```python
from build123d import *

# Parameters (mm, degrees)
BOSS_EXTRUDE1_DEPTH     = 3.175
CUT_EXTRUDE2_DEPTH      = 157.840117636
CUT_EXTRUDE2_DEPTH_BACK = 157.840117636
SKETCH3_R               = 1.25
CUT_EXTRUDE3_DEPTH      = 157.840117636
CUT_EXTRUDE3_DEPTH_BACK = 157.840117636
BOSS_EXTRUDE2_DEPTH     = 6.35
FILLET1_R               = 5
M6_CLEARANCE_HOLE1_D    = 6.6


with BuildPart() as part:
    # Sketch1 → Boss-Extrude1 (new, symmetric)
    with BuildSketch(Plane.XY):
        with BuildLine():
            Line((92.5, 126.5), (-92.5, 126.5))
            Line((-92.5, 126.5), (-92.5, 86.5))
            Line((-92.5, 86.5), (-42.012601066, -19.929660099))
            ThreePointArc((-42.012601066, -19.929660099), (0, -46.5), (42.012601066, -19.929660099))
            Line((42.012601066, -19.929660099), (92.5, 86.5))
            Line((92.5, 86.5), (92.5, 126.5))
        make_face()
    extrude(amount=BOSS_EXTRUDE1_DEPTH, both=True)

    # Sketch3 → Cut-Extrude2 (cut, two sides: drawn at the far end of the back side and taken through both)
    with BuildSketch(Plane(origin=(0, 0, -3.175), x_dir=(-1, 0, 0), z_dir=(0, 0, -1)).offset(-CUT_EXTRUDE2_DEPTH_BACK)):
        with Locations((17.440159599, -16.121517706)):
            Circle(SKETCH3_R)
        with Locations((22.282044228, -8.220280106)):
            Circle(SKETCH3_R)
        with Locations((9.943168767, -21.568400378)):
            Circle(SKETCH3_R)
        with Locations((0.932420624, -23.731689611)):
            Circle(SKETCH3_R)
        with Locations((-8.220280106, -22.282044228)):
            Circle(SKETCH3_R)
        with Locations((-16.121517706, -17.440159599)):
            Circle(SKETCH3_R)
        with Locations((-21.568400378, -9.943168767)):
            Circle(SKETCH3_R)
        with Locations((-23.731689611, -0.932420624)):
            Circle(SKETCH3_R)
        with Locations((-22.282044228, 8.220280106)):
            Circle(SKETCH3_R)
        with Locations((-17.440159599, 16.121517706)):
            Circle(SKETCH3_R)
        with Locations((-9.943168767, 21.568400378)):
            Circle(SKETCH3_R)
        with Locations((-0.932420624, 23.731689611)):
            Circle(SKETCH3_R)
        with Locations((8.220280106, 22.282044228)):
            Circle(SKETCH3_R)
        with Locations((16.121517706, 17.440159599)):
            Circle(SKETCH3_R)
        with Locations((21.568400378, 9.943168767)):
            Circle(SKETCH3_R)
        with Locations((23.731689611, 0.932420624)):
            Circle(SKETCH3_R)
    extrude(amount=CUT_EXTRUDE2_DEPTH + CUT_EXTRUDE2_DEPTH_BACK, mode=Mode.SUBTRACT)

    # Sketch4 → Cut-Extrude3 (cut, two sides: drawn at the far end of the back side and taken through both)
    with BuildSketch(Plane(origin=(0, 0, -3.175), x_dir=(-1, 0, 0), z_dir=(0, 0, -1)).offset(-CUT_EXTRUDE3_DEPTH_BACK)):
        with BuildLine():
            Line((-41.126950817, 21.698477285), (-73.85821292, 90.697419076))
            Line((-73.85821292, 90.697419076), (-73.85821292, 107.85821292))
            Line((-73.85821292, 107.85821292), (73.85821292, 107.85821292))
            Line((73.85821292, 107.85821292), (73.85821292, 90.697419076))
            Line((73.85821292, 90.697419076), (41.126950817, 21.698477285))
            ThreePointArc((41.126950817, 21.698477285), (0, 46.5), (-41.126950817, 21.698477285))
        make_face()
    extrude(amount=CUT_EXTRUDE3_DEPTH + CUT_EXTRUDE3_DEPTH_BACK, mode=Mode.SUBTRACT)

    # Sketch6 → Boss-Extrude2 (add)
    with BuildSketch(Plane.XY.offset(3.175)):
        Polygon((-32.71522073, 17.68327451), (0, 86.220686434), (32.71522073, 17.68327451), (49.538680905, 25.71368006), (10.328321936, 107.85821292), (-10.328321936, 107.85821292), (-49.538680905, 25.71368006), align=None)
    extrude(amount=-BOSS_EXTRUDE2_DEPTH)

    # Fillet1
    fillet1_edges = [part.edges().sort_by_distance(p)[0] for p in [
        (73.85821292, 90.697419076, 0),
        (73.85821292, 107.85821292, 0),
        (-73.85821292, 107.85821292, 0),
        (-73.85821292, 90.697419076, 0),
        (-46.275048201, 32.550893259, 0),
        (-21.466818467, 41.248341844, 0),
        (21.466818467, 41.248341844, 0),
        (0, 86.220686434, 0),
        (10.328321936, 107.85821292, 0),
        (-10.328321936, 107.85821292, 0),
        (46.275048201, 32.550893259, 0),
    ]]
    fillet(fillet1_edges, radius=FILLET1_R)

    # M6 Clearance Hole1 (through all)
    with Locations(Plane.XY.offset(3.175)):
        with Locations((83.17910646, 106.5), (-83.17910646, 106.5)):
            Hole(M6_CLEARANCE_HOLE1_D / 2)


solid = part.part
```
Model file for the job. Use its own axes, mm. A direction names the side the tool comes from. Coordinates: 2 decimals unless noted, no trailing zeros. Write each loop counter-clockwise with the first axis right and the second up, starting at its lowest first coordinate (ties: lowest second). Pieces come first, ordered by that corner, then holes. Notation, with made-up numbers: (-19.5, -2) - (13.5, -2) arc R27 ccw to (13.5, 25) - close; hole circle Ø11 at (19.25, 54). An arc over 180 degrees is marked (long way). One line per item, written item: value. Start each with the question number.
1. Slice it at A-A (x = -30). Write the cut outline in (y, z) (3 decimals).
2. Tool access for faces 4 (the flat face through (-92.5, 107, 0)), 5 (the flat face through (61.92, 65.53, 0.04)): list every direction of +Z, -Z, +X, -X, +Y, -Y with a clear straight run to the whole face (end or side of a thin tool).
3. Slice it at D-D (x = -77.5). Write the cut outline in (y, z) (3 decimals), plus the area to 3 significant figures.
4. Slice it at C-C (x = 28). Write the cut outline in (y, z) (3 decimals), plus the area to 3 significant figures.
5. Flat gauge pins, fed straight in: pin 1 (1.9 mm diameter, centred on x = 50.5, z = -1, fed in from -Y); pin 2 (1.5 mm diameter, centred on x = 17.44, y = 16.12, fed in from -Z) (3 decimals); pin 3 (3 mm diameter, centred on x = -39.5, z = 1, fed in from -Y); pin 4 (1 mm diameter, centred on y = 37, z = 1.5, fed in from +X). Where does each tip first touch, or does it go through?
6. Slice it at B-B (z = -1). Count the separate pieces of the cut face and the enclosed holes in it, plus the area to 3 significant figures.
7. Mould opens along X. For faces 1 (the flat face through (-1, 41, 3.175)), 2 (the flat face through (92.5, 106, 0)), 3 (the cylindrical face through (-15.52, 46.966, 0.044)) say: released by +X, released by -X, zero draft, split by the parting line, or undercut.
8. Probe line 1 (Y direction, x = -24, z = 2.25); line 2 (X direction, y = 85.5, z = -1.5); line 3 (X direction, y = 85, z = -3). List the from-to ranges inside material, lowest first. Write a range as from..to.
Answers below:
1. outline: (-35.528, -3.175) - (66.647, -3.175) - (66.647, 3.175) - (-35.528, 3.175) - close; (107.858, -3.175) - (126.5, -3.175) - (126.5, 3.175) - (107.858, 3.175) - close
2. face 4: +Z, -Z, -X, +Y, -Y
2. face 5: +Z, -Z
3. outline: (54.879, -3.175) - (126.5, -3.175) - (126.5, 3.175) - (54.879, 3.175) - close
3. area: 455 mm^2
4. outline: (-37.125, -3.175) - (70.837, -3.175) - (70.837, 3.175) - (-37.125, 3.175) - close; (107.858, -3.175) - (126.5, -3.175) - (126.5, 3.175) - (107.858, 3.175) - close
4. area: 804 mm^2
5. pin 1: stops at y = -4.04
5. pin 2: passes through
5. pin 3: stops at y = -26.8
5. pin 4: stops at x = 69.26
6. separate pieces: 1
6. enclosed holes: 21
6. area: 17,300 mm^2
7. face 1: zero draft
7. face 2: released by +X
7. face 3: undercut
8. line 1: y = -39.83..-0.29, 2.15..79.22, 107.86..126.5
8. line 2: x = -92.03..-71.39, -21..21, 71.39..92.03
8. line 3: x = -91.79..-71.16, -21.24..21.24, 71.16..91.79
